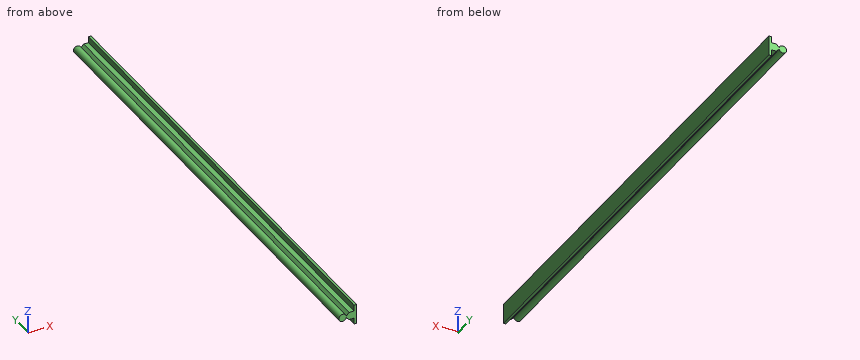
Autodesk Inventor part; units mm, degrees
ref_plane "YZ Plane" through (0, 0, 0) normal (1, 0, 0) x (0, 1, 0)
ref_plane "XZ Plane" through (0, 0, 0) normal (0, 1, 0) x (-1, 0, 0)
ref_plane "XY Plane" through (0, 0, 0) normal (0, 0, 1) x (1, 0, 0)
sketch "Sketch1" plane through (0, 0, 0) normal (0, 1, 0) x (-1, 0, 0)
  line L0 (-22.5, -6) -> (-22.5, 6)
  line L1 (-10.5, -6) -> (-5.8469, -1.3469)
  line L2 (-10.5, -6) -> (-3.9195, -6) construction
  line L3 (-10.5, 6) -> (-5.8469, 1.3469)
  arc A0 (-5.8469, -1.3469) -> (-5.8469, 1.3469) centre (-0.0057, 0) ccw
  line L4 (-22.5, 16) -> (-22.5, -16)
  line L5 (-22.5, -16) -> (-18.5, -16)
  line L6 (-18.5, 16) -> (-22.5, 16)
  line L7 (-18.5, -16) -> (-18.5, -6)
  line L8 (-18.5, 16) -> (-18.5, 6)
  line L9 (-10.5, 6) -> (-18.5, 6)
  line L10 (-10.5, -6) -> (-18.5, -6)
  point P0 (0, 0)
  dimension "d2" = 12
  dimension "d3" = 45
  dimension "d4" = 12
  dimension "d6" = 5.9944
  dimension "d7" = 32
  dimension "d8" = 4
  dimension "d10" = 0
extrude "Extrusion1" add sketch "Sketch1" along normal blind 800
properties part number "supportedRail_SBR12_800mm"
Part model, mm, in its own coordinate system. Round coordinates to 2 decimals unless told otherwise and drop trailing zeros. Write each loop counter-clockwise with the first axis right and the second up, starting at its lowest first coordinate (ties: lowest second). Pieces come first, ordered by that corner, then holes. Notation, with made-up numbers: M 74,59 L 110,59 A17 cw 110,66 Z; hole C 42,-9 d8. An arc over 180 degrees is marked long. Return JSON: item names as keys, results as strings. Group by question number.
(1) Saw through at A-A on y = 86. Write the cut outline in (x, z), then the cut area to 3 significant figures.
(2) Saw through at B-B on z = -11. Write the cut outline in (x, y), then the cut area to 3 significant figures.
(3) Drill centre lines: probe 1 along X at (y, z) = (258.5, -7.5); probe 2 along X at (y, z) = (42.5, -2.5); probe 3 along X at (y, z) = (507.5, 1.5). Where is each one in solid material? Low to high.
(4) Pin check, flat tips, straight feed: pin 1 Ø1.5 at (y, z) = (195.5, 10) entering from -X; pin 2 Ø1.5 at (x, z) = (16, 8.5) entering from +Y; pin 3 Ø2.5 at (x, y) = (13.5, 438) entering from -Z; pin 4 Ø8 at (y, z) = (260, -9.5) entering from -X. Stop position of each tip, or through.
Returned:
{
 "1": {"outline": "M 5.85,-1.35 L 10.5,-6 L 18.5,-6 L 18.5,-16 L 22.5,-16 L 22.5,16 L 18.5,16 L 18.5,6 L 10.5,6 L 5.85,1.35 A5.99 ccw long Z", "area": "371 mm²"},
 "2": {"outline": "M 18.5,0 L 22.5,0 L 22.5,800 L 18.5,800 Z", "area": "3,200 mm²"},
 "3": {"probe 1": "18.5 to 22.5", "probe 2": "-5.44 to 5.45, 7 to 22.5", "probe 3": "-5.8 to 5.81, 6 to 22.5"},
 "4": {"pin 1": "x = 18.5", "pin 2": "through", "pin 3": "z = -6", "pin 4": "x = -2.38"}
}
